```python
from build123d import *

# Parameters (mm, degrees)
EXTRUDE_1_DEPTH = 8


with BuildPart() as part:
    # Эскиз1 → Бобышка-Вытянуть1 (new body)
    with BuildSketch(Plane(origin=(0, 0, 0), x_dir=(1, 0, 0), z_dir=(0, 1, 0))):
        with BuildLine():
            Line((-25, -21.5), (15, -21.5))
            ThreePointArc((15, -21.5), (22.071067812, -18.571067812), (25, -11.5))
            Line((25, -11.5), (25, 21.5))
            Line((25, 21.5), (-25, 21.5))
            Line((-25, 21.5), (-25, -21.5))
        make_face()
    extrude(amount=EXTRUDE_1_DEPTH)


solid = part.part
```
Work out the finished part from the listing and answer in its coordinate system (mm). Round coordinates to 2 decimals unless told otherwise and drop trailing zeros. Write each loop counter-clockwise with the first axis right and the second up, starting at its lowest first coordinate (ties: lowest second). Pieces come first, ordered by that corner, then holes. Notation, with made-up numbers: (26, 65.25) -> (51, 65.25) arc R12 ccw to (51, 80.25) -> close; hole circle Ø4 at (-17.75, 47). An arc over 180 degrees is marked (long way). Write each question's results on one line, items separated by ' | '.
1) A flat-ended cylindrical pin translates along its axis: pin 1 (6 mm diameter, centred on x = 6.5, z = -2.5, fed in from -Y). Find the tip coordinate at first contact, or state that the pin passes through.
Findings:
pin 1: stops at y = 0
2) Consider line 1 along Z through (x, y) = (16, 5.5); line 2 along Z through (x, y) = (22, 2); line 3 along X through (y, z) = (4.25, 20.5). Determine where each line is inside the solid, lowest interval first. Write a range as [from, to].
Findings:
line 1: z = [-21.5, 21.45] | line 2: z = [-21.5, 18.64] | line 3: x = [-25, 19.36]
3) The part is cut by section A-A (x = 19). Write down the section's boundary in (y, z).
Findings:
outline: (0, -21.5) -> (8, -21.5) -> (8, 20.67) -> (0, 20.67) -> close
